Read the model definition and answer for the solid it produces. Units are mm, in the model's axes. A direction names the side the tool comes from. Coordinates: 2 decimals unless noted, no trailing zeros. Write each loop counter-clockwise with the first axis right and the second up, starting at its lowest first coordinate (ties: lowest second). Pieces come first, ordered by that corner, then holes. Notation, with made-up numbers: (-12.5, 0) -> (18.5, 0) arc R20 cw to (18.5, 29) -> close; hole circle Ø11 at (6, -13.75). An arc over 180 degrees is marked (long way). Answer in a Markdown table with one row per item. Add a question column.
Item 1: Which of the six approach directions +Z, -Z, +X, -X, +Y, -Y give full straight-line access (tool end or side, diameter ignored) to faces 1 (the face through (11.5, 7.2, 0.3)), 2 (the face through (6, 0.2, 0)), 3 (the face through (6, 6, 1.4))?
Item 2: For a pull along X with two mould halves and no side action, classify faces 4 (the face through (6, 6, 1)), 5 (the face through (12, 6.9, 0.3)), 6 (the face through (6, 0, 1)) as +X half, -X half, draft (parallel to the pull), parting line (faces both ways), or undercut.
Item 3: Given pin 1 Ø0.8 at (x, z) = (6.5, 0.5) entering from +Y; pin 2 Ø0.7 at (y, z) = (5, -0.5) entering from -X; pin 3 Ø0.6 at (x, z) = (0, -1) entering from -Y; pin 4 Ø2 at (x, y) = (6.5, 9.5) entering from -Z, each flat-ended and moving along its own axis, determine where each tip first touches the part or whether it passes through.
Item 4: Straight lines are drawn through the part: line 1 (X direction, y = 11.25, z = -0.3); line 2 (Z direction, x = 4.25, y = 4); line 3 (Y direction, x = 10.25, z = 0.5). For each, find the intervals that lie inside material, in ascending order. Write a range as from..to.
Item 5: Section C-C on y = 2 is taken. Write down the section's boundary in (x, z).
Item 6: Section B-B on z = 0.55 is taken. Write down the section's boundary in (x, y).
Item 7: Section D-D on x = 6.75 is taken. Write down the section's boundary in (y, z).
Item 8: Section A-A on z = -0.85 is taken. Write down the section's boundary in (x, y).
```python
from build123d import *

# Parameters (mm, degrees)
F1_DEPTH = 1.4
F3_DEPTH = 1
F4_W     = 0.5
F4_H     = 2
F5_DEPTH = 1.3
F6_R     = 0.5


with BuildPart() as f1:
    # F0 (on Top) → F1 (new body)
    with BuildSketch(Plane.XY):
        Polygon((0, 11.4), (0, 0), (12, 0), (12, 11.4), (10.8, 11.4), (10.8, 10), (2.4, 10), (2.4, 11.4), align=None)
    extrude(amount=F1_DEPTH)

    # F2 (on face) → F3 (cut)
    with BuildSketch(Plane(origin=(0, 0, 0), x_dir=(1, 0, 0), z_dir=(0, 0, -1))):
        Polygon((11.5, -0.5), (0.5, -0.5), (0.5, -11.4), (2.4, -11.4), (2.4, -10), (10.8, -10), (10.8, -11.4), (11.5, -11.4), align=None)
    extrude(amount=-F3_DEPTH, mode=Mode.SUBTRACT)

    # F4 (on face) → F5 (join)
    with BuildSketch(Plane(origin=(0, 0, 0), x_dir=(1, 0, 0), z_dir=(0, 0, -1))):
        with Locations((0.25, -10.4)):
            Rectangle(F4_W, F4_H)
        with Locations((11.75, -10.4)):
            Rectangle(F4_W, F4_H)
    extrude(amount=F5_DEPTH)

    # F6
    f6_edges = [f1.edges().sort_by_distance(p)[0] for p in [
        (10.8, 10, 1.2),
        (2.4, 10, 1.2),
    ]]
    fillet(f6_edges, radius=F6_R)


solid = f1.part
```
Results below:
| question | item | result |
|---|---|---|
| 1 | face 1 | -Z, +Y |
| 1 | face 2 | -Z, +X, -X, -Y |
| 1 | face 3 | +Z, +X, -X, +Y, -Y |
| 2 | face 4 | undercut |
| 2 | face 5 | +X half |
| 2 | face 6 | draft |
| 3 | pin 1 | stops at y = 0.5 |
| 3 | pin 2 | passes through |
| 3 | pin 3 | stops at y = 9.4 |
| 3 | pin 4 | stops at z = 1 |
| 4 | line 1 | x = 0..0.5, 11.5..12 |
| 4 | line 2 | z = 1..1.4 |
| 4 | line 3 | y = 0..0.5 |
| 5 | outline | (0, 0) -> (0.5, 0) -> (0.5, 1) -> (11.5, 1) -> (11.5, 0) -> (12, 0) -> (12, 1.4) -> (0, 1.4) -> close |
| 6 | outline | (0, 0) -> (12, 0) -> (12, 11.4) -> (11.5, 11.4) -> (11.5, 0.5) -> (0.5, 0.5) -> (0.5, 11.4) -> (0, 11.4) -> close |
| 7 | outline | (0, 0) -> (0.5, 0) -> (0.5, 1) -> (10, 1) -> (10, 1.4) -> (0, 1.4) -> close |
| 8 | outline | (0, 9.4) -> (0.5, 9.4) -> (0.5, 11.4) -> (0, 11.4) -> close; (11.5, 9.4) -> (12, 9.4) -> (12, 11.4) -> (11.5, 11.4) -> close |
